Verification items for the finished model (mm, model axes). A direction names the side the tool comes from. Round coordinates to 2 decimals unless told otherwise and drop trailing zeros. Order: outer loops, then holes, each group sorted by start corner. A loop starts at its lowest first (then second) coordinate and runs counter-clockwise, first axis right, second up. Notation, with made-up numbers: (-12.75, -21.5) -> (-8.75, -21.5) arc R10 cw to (-8.75, -8.5) -> close; hole circle Ø3 at (-7.5, -15). An arc over 180 degrees is marked (long way). Write item = value, one per line. Start each with the question number.
from build123d import *

# Parameters (mm, degrees)
SKETCH1_W                                           = 25
SKETCH1_H                                           = 38
BOSS_EXTRUDE1_DEPTH                                 = 17
CUT_EXTRUDE3_DEPTH                                  = 3.7
CUT_EXTRUDE4_DEPTH                                  = 1.7
CBORE_FOR_6_BINDING_HEAD_MACHINE_SCREW1_D           = 3.7973
CBORE_FOR_6_BINDING_HEAD_MACHINE_SCREW1_CBORE_D     = 7.9375
CBORE_FOR_6_BINDING_HEAD_MACHINE_SCREW1_CBORE_DEPTH = 2.2098


with BuildPart() as part:
    # Sketch1 → Boss-Extrude1 (new body)
    with BuildSketch(Plane(origin=(0, 0, 0), x_dir=(1, 0, 0), z_dir=(0, 1, 0))):
        with Locations((-18481.446731235, 11298.191283293)):
            Rectangle(SKETCH1_W, SKETCH1_H)
    extrude(amount=BOSS_EXTRUDE1_DEPTH)

    # Sketch2 → Cut-Extrude3 (cut)
    with BuildSketch(Plane(origin=(0, 17, 0), x_dir=(1, 0, 0), z_dir=(0, 1, 0))):
        with BuildLine():
            Line((-18493.946731235, 11291.191283293), (-18489.946731235, 11291.191283293))
            ThreePointArc((-18489.946731235, 11291.191283293), (-18488.532517672, 11291.777069731), (-18487.946731235, 11293.191283293))
            Line((-18487.946731235, 11293.191283293), (-18487.946731235, 11303.191283293))
            ThreePointArc((-18487.946731235, 11303.191283293), (-18488.532517672, 11304.605496855), (-18489.946731235, 11305.191283293))
            Line((-18489.946731235, 11305.191283293), (-18493.946731235, 11305.191283293))
            Line((-18493.946731235, 11305.191283293), (-18493.946731235, 11291.191283293))
        make_face()
    extrude(amount=-CUT_EXTRUDE3_DEPTH, mode=Mode.SUBTRACT)

    # Sketch2<6> → Cut-Extrude4 (cut)
    with BuildSketch(Plane(origin=(0, 17, 0), x_dir=(1, 0, 0), z_dir=(0, 1, 0))):
        with BuildLine():
            Line((-18475.446731235, 11301.191283293), (-18475.446731235, 11295.191283293))
            ThreePointArc((-18475.446731235, 11295.191283293), (-18474.860944797, 11293.777069731), (-18473.446731235, 11293.191283293))
            Line((-18473.446731235, 11293.191283293), (-18468.946731235, 11293.191283293))
            Line((-18468.946731235, 11293.191283293), (-18468.946731235, 11303.191283293))
            Line((-18468.946731235, 11303.191283293), (-18473.446731235, 11303.191283293))
            ThreePointArc((-18473.446731235, 11303.191283293), (-18474.860944797, 11302.605496855), (-18475.446731235, 11301.191283293))
        make_face()
    extrude(amount=-CUT_EXTRUDE4_DEPTH, mode=Mode.SUBTRACT)

    # CBORE for #6 Binding Head Machine Screw1 (through all)
    with Locations(Plane(origin=(0, 17, 0), x_dir=(1, 0, 0), z_dir=(0, 1, 0))):
        with Locations((-18488.946731235, 11310.191283293), (-18473.946731235, 11310.191283293), (-18473.946731235, 11286.191283293), (-18488.946731235, 11286.191283293)):
            CounterBoreHole(CBORE_FOR_6_BINDING_HEAD_MACHINE_SCREW1_D / 2, CBORE_FOR_6_BINDING_HEAD_MACHINE_SCREW1_CBORE_D / 2, CBORE_FOR_6_BINDING_HEAD_MACHINE_SCREW1_CBORE_DEPTH)


solid = part.part
(1) Depth check by flat-ended pin: pin 1 (2.5 mm diameter, centred on x = -18490.5, z = -11288, fed in from +Y); pin 2 (3 mm diameter, centred on x = -18473, z = -11300, fed in from +Y); pin 3 (4 mm diameter, centred on y = 16, z = -11297.5, fed in from -X). Enter the tip coordinate at first touch or a pass-through.
(2) Cross-section at D-D (z = -11298). Enter the section's corners in (x, y), and give its area (3 significant figures).
(3) Scan lines: line 1 along X through (y, z) = (16.25, -11286); line 2 along X through (y, z) = (11.25, -11286); line 3 along Z through (x, y) = (-18475.5, 2.75). Record each from-to range of solid material in increasing order. Write a range as from..to.
(4) Cross-section at A-A (z = -11287). Enter the section's corners in (x, y), and give its area (3 significant figures).
(5) Set-up check for faces 1 (the cylindrical face through (-18476.872, 15.911, -11288.874)), 2 (the cylindrical face through (-18474.845, 16.162, -11302.621)), 3 (the flat face through (-18492, 15, -11291.191)), 4 (the cylindrical face through (-18472.44, 7.292, -11309.036)): record each of +Z, -Z, +X, -X, +Y, -Y from which the full face is reachable in a straight line by a thin tool's end or side.
(6) Cross-section at C-C (y = 16.25). Enter the section's corners in (x, z).
(7) Cross-section at B-B (x = -18489.5). Enter the section's corners in (y, z), and give its area (3 significant figures).
(8) Draft check along X on faces 5 (the flat face through (-18482, 0, -11298)), 6 (the cylindrical face through (-18488.55, 15.18, -11291.76)), 7 (the cylindrical face through (-18487.44, 7.292, -11285.036)). Enter one of: +X half, -X half, draft (parallel to the pull), parting line (faces both ways), or undercut.
Outcome:
q1.pin_1 = 14.79
q1.pin_2 = 15.3
q1.pin_3 = -18487.95
q2.outline = (-18493.95, 0) -> (-18468.95, 0) -> (-18468.95, 15.3) -> (-18475.45, 15.3) -> (-18475.45, 17) -> (-18487.95, 17) -> (-18487.95, 13.3) -> (-18493.95, 13.3) -> close
q2.area = 392 mm^2
q3.line_1 = -18493.95..-18492.91, -18484.98..-18477.91, -18469.98..-18468.95
q3.line_2 = -18493.95..-18490.84, -18487.06..-18475.84, -18472.06..-18468.95
q3.line_3 = -11317.19..-11311.28, -11309.1..-11287.28, -11285.1..-11279.19
q4.outline = (-18493.95, 0) -> (-18490.66, 0) -> (-18490.66, 14.79) -> (-18492.83, 14.79) -> (-18492.83, 17) -> (-18493.95, 17) -> close; (-18487.23, 0) -> (-18475.66, 0) -> (-18475.66, 14.79) -> (-18477.83, 14.79) -> (-18477.83, 17) -> (-18485.06, 17) -> (-18485.06, 14.79) -> (-18487.23, 14.79) -> close; (-18472.23, 0) -> (-18468.95, 0) -> (-18468.95, 17) -> (-18470.06, 17) -> (-18470.06, 14.79) -> (-18472.23, 14.79) -> close
q4.area = 289 mm^2
q5.face_1 = +Y
q5.face_2 = +X, +Y
q5.face_3 = -X, +Y
q5.face_4 = +Y, -Y
q6.outline = (-18493.95, -11317.19) -> (-18468.95, -11317.19) -> (-18468.95, -11303.19) -> (-18473.45, -11303.19) arc R2 cw to (-18475.45, -11301.19) -> (-18475.45, -11295.19) arc R2 cw to (-18473.45, -11293.19) -> (-18468.95, -11293.19) -> (-18468.95, -11279.19) -> (-18493.95, -11279.19) -> (-18493.95, -11291.19) -> (-18489.95, -11291.19) arc R2 cw to (-18487.95, -11293.19) -> (-18487.95, -11303.19) arc R2 cw to (-18489.95, -11305.19) -> (-18493.95, -11305.19) -> close; hole circle Ø7.94 at (-18488.95, -11310.19); hole circle Ø7.94 at (-18488.95, -11286.19); hole circle Ø7.94 at (-18473.95, -11310.19); hole circle Ø7.94 at (-18473.95, -11286.19)
q7.outline = (0, -11317.19) -> (17, -11317.19) -> (17, -11314.12) -> (14.79, -11314.12) -> (14.79, -11312.01) -> (0, -11312.01) -> close; (0, -11308.38) -> (14.79, -11308.38) -> (14.79, -11306.26) -> (17, -11306.26) -> (17, -11305.14) -> (13.3, -11305.14) -> (13.3, -11291.24) -> (17, -11291.24) -> (17, -11290.12) -> (14.79, -11290.12) -> (14.79, -11288.01) -> (0, -11288.01) -> close; (0, -11284.38) -> (14.79, -11284.38) -> (14.79, -11282.26) -> (17, -11282.26) -> (17, -11279.19) -> (0, -11279.19) -> close
q7.area = 452 mm^2
q8.face_5 = draft
q8.face_6 = -X half
q8.face_7 = undercut
